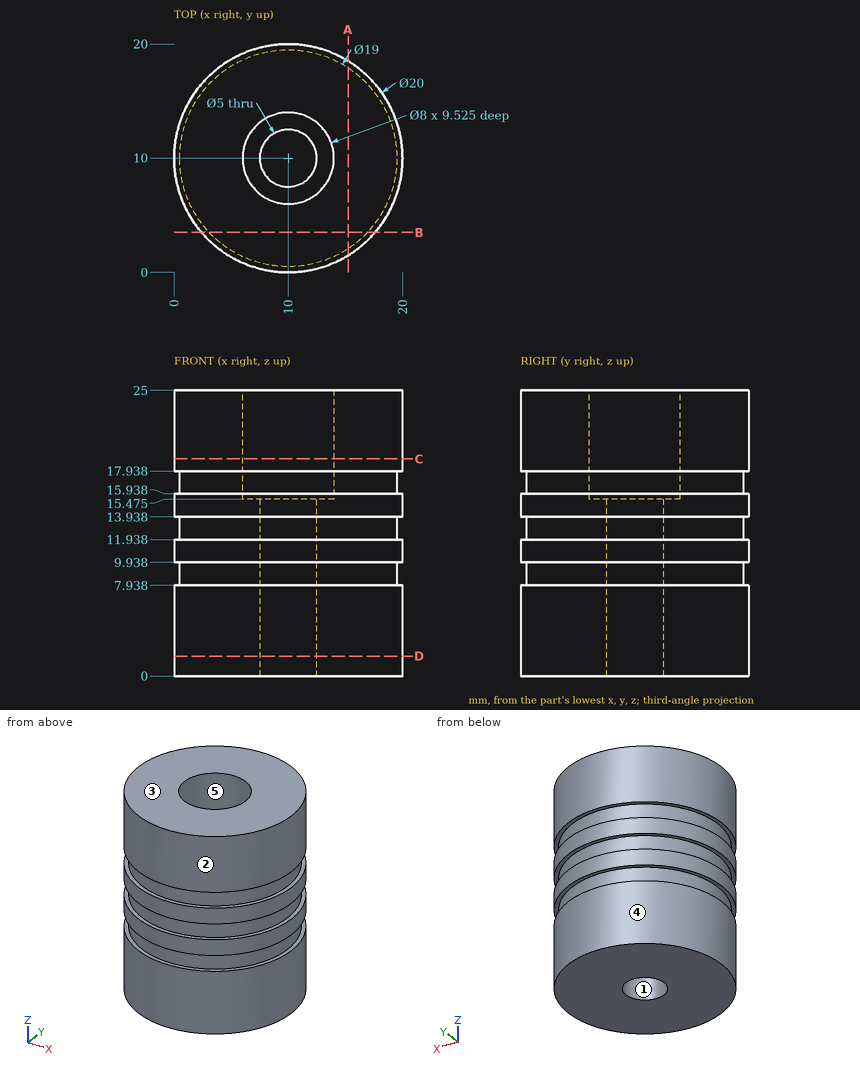
Drawing for the job (mm, zero at the part's lowest x, y, z). A direction names the side the tool comes from. Round coordinates to 2 decimals unless told otherwise and drop trailing zeros. Loops run counter-clockwise (first coordinate to the right, second up) from the corner with the lowest first, then second, coordinate; pieces in that order, holes last. Notation, with made-up numbers: (20, -38) - (73, -38) arc R34 cw to (73, -1) - close; hole circle Ø3 at (-11.5, 78). An arc over 180 degrees is marked (long way). Return JSON: item names as keys, results as strings. Group by question number.
Q1. Band-saw the part on C-C on z = 19. Give the cut face in (x, y), plus the area to 3 significant figures.
Q2. Two-plate mould, pull along Y, no slides. Class the marked faces 1, 2 and 3: +Y half, -Y half, draft (parallel to the pull), parting line (faces both ways), or undercut.
Q3. Band-saw the part on A-A on x = 15.25. Give the cut face in (y, z).
Q4. Band-saw the part on D-D on z = 1.75. Give the cut face in (x, y).
Q5. Flat gauge pins, fed straight in: pin 1 Ø10 at (x, z) = (16.5, 3) entering from -Y; pin 2 Ø6.5 at (x, y) = (10, 10) entering from +Z (1 decimal); pin 3 Ø1.5 at (x, z) = (14.5, 12) entering from +Y. Where does each tip first touch, or does it go through?
Q6. Band-saw the part on B-B on y = 3.5. Give the cut face in (x, z).
Q7. Drill centre lines: line 1 along Y through (x, z) = (10, 5.5); line 2 along Y through (x, z) = (10, 21.25); line 3 along Z through (x, y) = (10.25, 13.5) (1 decimal). Where is each one in solid material? Low to high. Write a range as [from, to].
Q8. Tool access for the marked faces 4 and 5: list every direction of +Z, -Z, +X, -X, +Y, -Y with a clear straight run to the whole face (end or side of a thin tool).
Solutions:
{
 "1": {"outline": "circle Ø20 at (10, 10); hole circle Ø8 at (10, 10)", "area": "264 mm^2"},
 "2": {"face 1": "undercut", "face 2": "parting line", "face 3": "draft"},
 "3": {"outline": "(1.49, 0) - (18.51, 0) - (18.51, 7.94) - (17.92, 7.94) - (17.92, 9.94) - (18.51, 9.94) - (18.51, 11.94) - (17.92, 11.94) - (17.92, 13.94) - (18.51, 13.94) - (18.51, 15.94) - (17.92, 15.94) - (17.92, 17.94) - (18.51, 17.94) - (18.51, 25) - (1.49, 25) - (1.49, 17.94) - (2.08, 17.94) - (2.08, 15.94) - (1.49, 15.94) - (1.49, 13.94) - (2.08, 13.94) - (2.08, 11.94) - (1.49, 11.94) - (1.49, 9.94) - (2.08, 9.94) - (2.08, 7.94) - (1.49, 7.94) - close"},
 "4": {"outline": "circle Ø20 at (10, 10); hole circle Ø5 at (10, 10)"},
 "5": {"pin 1": "stops at y = 0.11", "pin 2": "stops at z = 15.5", "pin 3": "stops at y = 19.27"},
 "6": {"outline": "(2.4, 0) - (17.6, 0) - (17.6, 7.94) - (16.93, 7.94) - (16.93, 9.94) - (17.6, 9.94) - (17.6, 11.94) - (16.93, 11.94) - (16.93, 13.94) - (17.6, 13.94) - (17.6, 15.94) - (16.93, 15.94) - (16.93, 17.94) - (17.6, 17.94) - (17.6, 25) - (2.4, 25) - (2.4, 17.94) - (3.07, 17.94) - (3.07, 15.94) - (2.4, 15.94) - (2.4, 13.94) - (3.07, 13.94) - (3.07, 11.94) - (2.4, 11.94) - (2.4, 9.94) - (3.07, 9.94) - (3.07, 7.94) - (2.4, 7.94) - close"},
 "7": {"line 1": "y = [0, 7.5], [12.5, 20]", "line 2": "y = [0, 6], [14, 20]", "line 3": "z = [0, 15.5]"},
 "8": {"face 4": "+Z, -Z", "face 5": "+Z"}
}
